Could you check a few things on this model? Use its own coordinates, in mm. Coordinates: 2 decimals unless noted, no trailing zeros. Loops run counter-clockwise (first coordinate to the right, second up) from the corner with the lowest first, then second, coordinate; pieces in that order, holes last.
1) Imagine slicing it at B-B on y = 6. Please give me the cut outline in (x, z).
2) If I drill on line 1 along Y through (x, z) = (-1.5, 202); line 2 along X through (y, z) = (1, 204); line 3 along Z through (x, y) = (-20, -11.5), over which ranges is the centre line in solid material (lowest first)?
3) Imagine slicing it at C-C on z = 351. Please give me the cut outline in (x, y) (3 decimals), plus the area to 3 significant figures.
4) Imagine slicing it at A-A on x = 8. Please give me the cut outline in (y, z).
5) Thinking about a two-plate mould opening in X: for faces 1 (the face through (16, -16, 450)), 2 (the face through (-5.149, -23.185, 221.85)), 3 (the face through (-4.8, -21.7, 221.8)), which applies, released by +X, released by -X, zero draft, split by the parting line, or undercut?
6) Will these pins go through, and if not, where does the flat tip stop? P1, Ø12, axis at y = -9.5, z = 168.5, coming from the -X side; P2, Ø2, axis at y = -5.5, z = 230.5, coming from the +X side; P3, Ø6, axis at y = -11, z = 270, coming from the -X side.
```python
from build123d import *

# Parameters (mm, degrees)
SKETCH1_R           = 23.75
SKETCH1_R_2         = 22.225
BOSS_EXTRUDE1_DEPTH = 450
CUT_EXTRUDE1_START  = -77.970542
SKETCH2_W           = 4.52920266
SKETCH2_H           = 30
CUT_EXTRUDE1_DEPTH  = 1.720542
CIRPATTERN2_COUNT   = 3


with BuildPart() as part:
    # Sketch1 → Boss-Extrude1 (new body)
    with BuildSketch(Plane.XY):
        Circle(SKETCH1_R)
        Circle(SKETCH1_R_2, mode=Mode.SUBTRACT)
    extrude(amount=BOSS_EXTRUDE1_DEPTH)

    # Sketch2 → Cut-Extrude1 (cut)
    with BuildSketch(Plane(origin=(0, 100, 0), x_dir=(1, 0, 0), z_dir=(0, 1, 0)).offset(CUT_EXTRUDE1_START)):
        with Locations((-0.67710133, -415.7565327)):
            Rectangle(SKETCH2_W, SKETCH2_H)
    cut_extrude1 = extrude(amount=CUT_EXTRUDE1_DEPTH, mode=Mode.SUBTRACT)

    # CirPattern2: Cut-Extrude1 ×3 about axis
    cirpattern2_axis = Axis((0, 0, 0), (0, 0, 1))
    for i in range(1, CIRPATTERN2_COUNT):
        add(cut_extrude1.rotate(cirpattern2_axis, i * 360 / CIRPATTERN2_COUNT), mode=Mode.SUBTRACT)


solid = part.part
```
Filled in:
1. outline: (-22.98, 0) - (-21.4, 0) - (-21.4, 450) - (-22.98, 450) - close; (21.4, 0) - (22.98, 0) - (22.98, 450) - (21.4, 450) - close
2. line 1: y = -23.7 to -22.17, 22.17 to 23.7
2. line 2: x = -23.73 to -22.2, 22.2 to 23.73
2. line 3: z = 0 to 400.76, 430.76 to 450
3. outline: circle Ø47.5 at (0, 0); hole circle Ø44.45 at (0, 0)
3. area: 220 mm2
4. outline: (-22.36, 0) - (-20.74, 0) - (-20.74, 450) - (-22.36, 450) - close; (20.74, 0) - (22.36, 0) - (22.36, 450) - (20.74, 450) - close
5. face 1: zero draft
5. face 2: split by the parting line
5. face 3: undercut
6. P1: stops at x = -23.49
6. P2: stops at x = 23.32
6. P3: stops at x = -22.36
